For this review, take the finished solid that the model builds, in its own axes (mm). Round coordinates to 2 decimals unless told otherwise and drop trailing zeros. Write each loop counter-clockwise with the first axis right and the second up, starting at its lowest first coordinate (ties: lowest second). Pieces come first, ordered by that corner, then holes.
from build123d import *

# Parameters (mm, degrees)
SKETCH1_R           = 2.75
BOSS_EXTRUDE1_DEPTH = 2
SKETCH2_R           = 2.55
BOSS_EXTRUDE2_DEPTH = 12
SKETCH3_R           = 2.75
BOSS_EXTRUDE3_DEPTH = 2
SKETCH4_R           = 0.35
BOSS_EXTRUDE4_DEPTH = 5
SKETCH5_R           = 0.35
BOSS_EXTRUDE5_DEPTH = 5
FILLET1_R           = 0.2
FILLET2_R           = 0.7


with BuildPart() as part:
    # Sketch1 → Boss-Extrude1 (new body)
    with BuildSketch(Plane.XY.offset(8)):
        Circle(SKETCH1_R)
    extrude(amount=-BOSS_EXTRUDE1_DEPTH)

    # Sketch2 → Boss-Extrude2 (add)
    with BuildSketch(Plane(origin=(0, 0, 6), x_dir=(-1, 0, 0), z_dir=(0, 0, -1))):
        Circle(SKETCH2_R)
    extrude(amount=BOSS_EXTRUDE2_DEPTH)

    # Sketch3 → Boss-Extrude3 (add)
    with BuildSketch(Plane.XY.offset(-6)):
        Circle(SKETCH3_R)
    extrude(amount=-BOSS_EXTRUDE3_DEPTH)

    # Sketch4 → Boss-Extrude4 (add)
    with BuildSketch(Plane.XY.offset(8)):
        Circle(SKETCH4_R)
    extrude(amount=BOSS_EXTRUDE4_DEPTH)

    # Sketch5 → Boss-Extrude5 (add)
    with BuildSketch(Plane(origin=(0, 0, -8), x_dir=(-1, 0, 0), z_dir=(0, 0, -1))):
        Circle(SKETCH5_R)
    extrude(amount=BOSS_EXTRUDE5_DEPTH)

    # Fillet1
    fillet1_edges = [part.edges().sort_by_distance(p)[0] for p in [
        (-2.75, 0, 8),
        (-2.75, 0, -8),
    ]]
    fillet(fillet1_edges, radius=FILLET1_R)

    # Fillet2
    fillet2_edges = [part.edges().sort_by_distance(p)[0] for p in [
        (-0.35, 0, 8),
        (0.35, 0, -8),
    ]]
    fillet(fillet2_edges, radius=FILLET2_R)


solid = part.part
(1) We need section D-D, the plane z = -9.75. Give the boundary of the cut face in (x, y), and give its area (3 significant figures).
Geometry check:
outline: circle Ø0.7 at (0, 0)
area: 0.385 mm2
(2) Mouldability with a two-part tool opening along Z and no side actions: class faces 1 (the face through (-0.596, -2.685, -6.887)), 2 (the face through (-1.18, -2.26, 0.08)), 3 (the face through (1, -1, -8)), 4 (the face through (1, -1, 8)) as pulls with the +Z half, pulls with the -Z half, needs draft (parallel to the pull), parting line crosses it, or undercut.
Geometry check:
face 1: needs draft
face 2: undercut
face 3: pulls with the -Z half
face 4: pulls with the +Z half
(3) For pin 1 Ø1.5 at (x, y) = (-1, 1.5) entering from +Z; pin 2 Ø1.5 at (y, z) = (-1, -2) entering from -X; pin 3 Ø1 at (x, z) = (0, 4.5) entering from +Y, all flat-tipped, find the tip position at first contact; note any pin that passes through.
Geometry check:
pin 1: stops at z = 8
pin 2: stops at x = -2.54
pin 3: stops at y = 2.55
(4) For line 1 along Z through (x, y) = (1.35, 1.9); line 2 along Y through (x, z) = (0.1, 5); line 3 along Y through (x, z) = (-1, -2.25), list the stretches that pass through material, from the lowest coordinate up.
Geometry check:
line 1: z = -8 to 8
line 2: y = -2.55 to 2.55
line 3: y = -2.35 to 2.35
(5) We need section C-C, the plane z = 4.5. Give the boundary of the cut face in (x, y).
Geometry check:
outline: circle Ø5.1 at (0, 0)
(6) We need section A-A, the plane y = 0. Give the boundary of the cut face in (x, z), and give its area (3 significant figures).
Geometry check:
outline: (-2.75, -7.8) arc R0.2 ccw to (-2.55, -8) - (-1.05, -8) arc R0.7 cw to (-0.35, -8.7) - (-0.35, -13) - (0.35, -13) - (0.35, -8.7) arc R0.7 cw to (1.05, -8) - (2.55, -8) arc R0.2 ccw to (2.75, -7.8) - (2.75, -6) - (2.55, -6) - (2.55, 6) - (2.75, 6) - (2.75, 7.8) arc R0.2 ccw to (2.55, 8) - (1.05, 8) arc R0.7 cw to (0.35, 8.7) - (0.35, 13) - (-0.35, 13) - (-0.35, 8.7) arc R0.7 cw to (-1.05, 8) - (-2.55, 8) arc R0.2 ccw to (-2.75, 7.8) - (-2.75, 6) - (-2.55, 6) - (-2.55, -6) - (-2.75, -6) - close
area: 90.6 mm2
